Geometry check sheet. Reference: drawing and pictorial views, mm from the part's lowest x, y, z. Round coordinates to 2 decimals unless told otherwise and drop trailing zeros. Order: outer loops, then holes, each group sorted by start corner. A loop starts at its lowest first (then second) coordinate and runs counter-clockwise, first axis right, second up. Notation, with made-up numbers: (50.25, 60) -> (59.25, 60) arc R15 ccw to (59.25, 76) -> close; hole circle Ø5 at (18, 27). An arc over 180 degrees is marked (long way). Put each result on its own line as item: value.
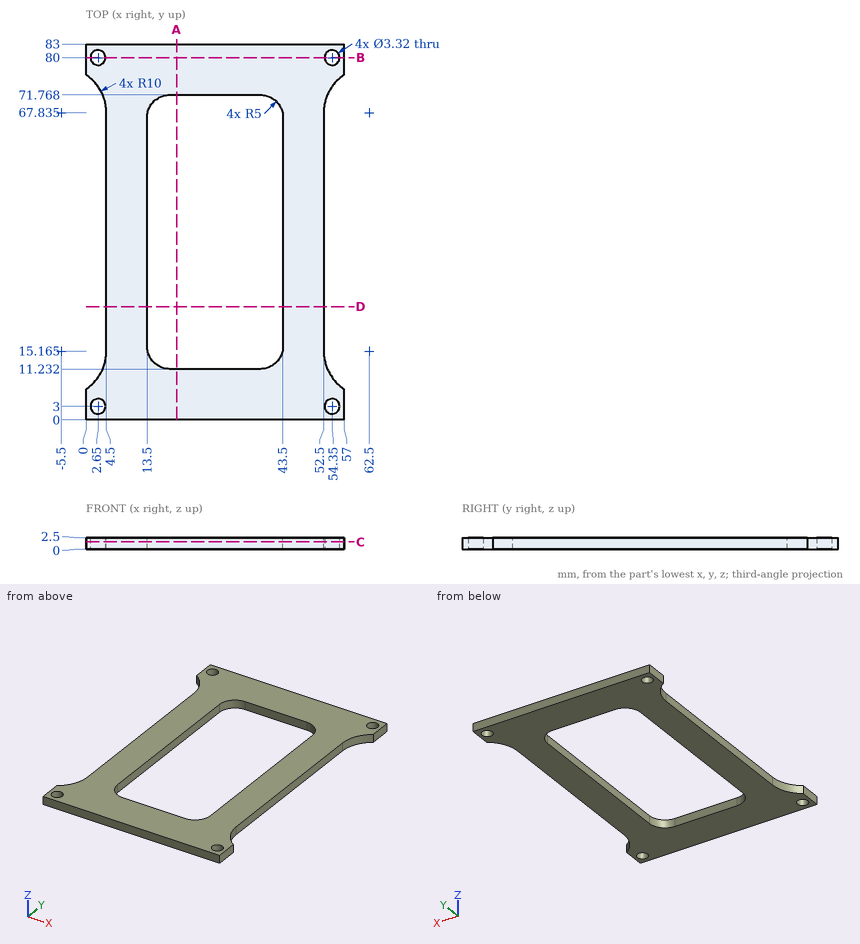
Item 1: Sectioned sample at C-C, the plane z = 1.6. Give the number of separate pieces and of enclosed holes in the cut face, then the cut area to 3 significant figures.
Geometry check:
separate pieces: 1
enclosed holes: 5
area: 2,320 mm2
Item 2: Sectioned sample at B-B, the plane y = 80. Record the boundary of the cut face in (x, z).
Geometry check:
outline: (0, 0) -> (0.99, 0) -> (0.99, 2.5) -> (0, 2.5) -> close; (4.31, 0) -> (52.69, 0) -> (52.69, 2.5) -> (4.31, 2.5) -> close; (56.01, 0) -> (57, 0) -> (57, 2.5) -> (56.01, 2.5) -> close
Item 3: Sectioned sample at A-A, the plane x = 20. Record the boundary of the cut face in (y, z).
Geometry check:
outline: (0, 0) -> (11.23, 0) -> (11.23, 2.5) -> (0, 2.5) -> close; (71.77, 0) -> (83, 0) -> (83, 2.5) -> (71.77, 2.5) -> close
Item 4: Material ranges on line 1 along X through (y, z) = (63, 2.05); line 2 along X through (y, z) = (80, 0.55); line 3 along Y through (x, z) = (28.5, 1), recorded low to high.
Geometry check:
line 1: 4.5 to 13.5, 43.5 to 52.5
line 2: 0 to 0.99, 4.31 to 52.69, 56.01 to 57
line 3: 0 to 11.23, 71.77 to 83
Item 5: Sectioned sample at D-D, the plane y = 25. Record the boundary of the cut face in (x, z), then the cut area to 3 significant figures.
Geometry check:
outline: (4.5, 0) -> (13.5, 0) -> (13.5, 2.5) -> (4.5, 2.5) -> close; (43.5, 0) -> (52.5, 0) -> (52.5, 2.5) -> (43.5, 2.5) -> close
area: 45.0 mm2
Item 6: Depth check by flat-ended pin: pin 1 Ø1.2 at (y, z) = (54, 1) entering from +X; pin 2 Ø1 at (y, z) = (13, 2) entering from -X; pin 3 Ø1.2 at (y, z) = (52, 0.5) entering from -X; pin 4 Ø6 at (x, y) = (47, 43) entering from -Z. Enter the tip coordinate at first touch or a pass-through.
Geometry check:
pin 1: x = 52.5
pin 2: x = 4.14
pin 3: x = 4.5
pin 4: z = 0
